from build123d import *

# Parameters (mm, degrees)
F1_DEPTH = 12.7
F2_DEPTH = 31.75
F3_R     = 12.7


with BuildPart() as f1:
    # F0 (on Right) → F1 (new body, symmetric)
    with BuildSketch(Plane.YZ):
        with BuildLine():
            ThreePointArc((31.059256, -22.06655), (36.29716, -11.581285), (38.1, 0))
            ThreePointArc((38.1, 0), (-11.489227, 36.326405), (-31.170744, -21.908782))
            Line((-31.170744, -21.908782), (31.059256, -21.908782))
            Line((31.059256, -21.908782), (31.059256, -22.06655))
        make_face()
        with BuildLine():
            Line((31.059256, -174.308782), (31.059256, -22.06655))
            ThreePointArc((31.059256, -22.06655), (17.476763, -33.855173), (0, -38.1))
            Line((0, -38.1), (-31.170744, -49.680229))
            Line((-31.170744, -49.680229), (-31.170744, -174.308782))
            Line((-31.170744, -174.308782), (31.059256, -174.308782))
        make_face()
        with BuildLine():
            Line((31.059256, -21.908782), (-31.170744, -21.908782))
            ThreePointArc((-31.170744, -21.908782), (-17.562537, -33.810757), (0, -38.1))
            ThreePointArc((0, -38.1), (17.476763, -33.855173), (31.059256, -22.06655))
            Line((31.059256, -22.06655), (31.059256, -21.908782))
        make_face()
    extrude(amount=F1_DEPTH, both=True)

    # F0 (on Right) → F2 (join, symmetric)
    with BuildSketch(Plane.YZ):
        with BuildLine():
            Line((31.059256, -174.308782), (31.059256, -22.06655))
            ThreePointArc((31.059256, -22.06655), (17.476763, -33.855173), (0, -38.1))
            Line((0, -38.1), (-31.170744, -49.680229))
            Line((-31.170744, -49.680229), (-31.170744, -174.308782))
            Line((-31.170744, -174.308782), (31.059256, -174.308782))
        make_face()
    extrude(amount=F2_DEPTH, both=True)

    # F3
    f3_edges = [f1.edges().sort_by_distance(p)[0] for p in [
        (31.75, -31.170744, -111.994506),
        (31.75, 31.059256, -98.187666),
        (-31.75, -31.170744, -111.994506),
        (-31.75, 31.059256, -98.187666),
    ]]
    fillet(f3_edges, radius=F3_R)


solid = f1.part
Read the model definition and answer for the solid it produces. Units are mm, in the model's axes. A direction names the side the tool comes from. Give positions to 0.01 mm unless a question says otherwise; leave off trailing zeros. Loops run counter-clockwise (first coordinate to the right, second up) from the corner with the lowest first, then second, coordinate; pieces in that order, holes last. Notation, with made-up numbers: (87.25, 52) -> (128.25, 52) arc R16 cw to (128.25, 80) -> close; hole circle Ø6 at (-38, 61.25). An arc over 180 degrees is marked (long way). Use a Markdown table: item, result.
Q1. Find the intervals of material crossed by line 1 along Y through (x, z) = (-14.5, -116); line 2 along X through (y, z) = (-34, 3.5); line 3 along Z through (x, y) = (-4.5, 1), in increasing order.
Solved:
| item | result |
|---|---|
| line 1 | y = -31.17 to 31.06 |
| line 2 | x = -12.7 to 12.7 |
| line 3 | z = -174.31 to 38.09 |
Q2. Section C-C, the plane y = -24 is taken. Determine the outline of the cut face in (x, z).
Solved:
| item | result |
|---|---|
| outline | (-30.48, -174.31) -> (30.48, -174.31) -> (30.48, -47.02) -> (-30.48, -47.02) -> close; (-12.7, -29.59) -> (12.7, -29.59) -> (12.7, 29.59) -> (-12.7, 29.59) -> close |
Q3. Section D-D, the plane y = 16 is taken. Determine the outline of the cut face in (x, z), then the cut area to 3 significant figures.
Solved:
| item | result |
|---|---|
| outline | (-31.75, -174.31) -> (31.75, -174.31) -> (31.75, -34.58) -> (12.7, -34.58) -> (12.7, 34.58) -> (-12.7, 34.58) -> (-12.7, -34.58) -> (-31.75, -34.58) -> close |
| area | 10,600 mm^2 |
Q4. A tool of negligible diameter and unlimited length cuts with its end or side. For faces 1 (the face through (-12.7, -1, 1)), 2 (the face through (0, -31.171, -111)), 3 (the face through (0, 31.059, -99)), 4 (the face through (12.7, -1, 1)), from which of +Z, -Z, +X, -X, +Y, -Y can it reach the whole face along a straight path? Write none if from no direction.
Solved:
| item | result |
|---|---|
| face 1 | +Z, -X, -Y |
| face 2 | -Z, +X, -X, -Y |
| face 3 | -Z, +X, -X, +Y |
| face 4 | +Z, +X, -Y |
Q5. Each of these flat-tipped pins is pushed along its axis until it touches: pin 1 (10 mm diameter, centred on x = -20.5, z = -75.5, fed in from -Y); pin 2 (1.5 mm diameter, centred on y = 22.5, z = -20.5, fed in from -X); pin 3 (19 mm diameter, centred on x = 5.5, z = -130, fed in from +Y). Where does it stop, or does it pass through?
Solved:
| item | result |
|---|---|
| pin 1 | stops at y = -31.17 |
| pin 2 | stops at x = -12.7 |
| pin 3 | stops at y = 31.06 |
Q6. Section B-B, the plane z = -128.5 is taken. Determine the outline of the cut face in (x, y), then the cut area to 3 significant figures.
Solved:
| item | result |
|---|---|
| outline | (-31.75, -18.47) arc R12.7 ccw to (-19.05, -31.17) -> (19.05, -31.17) arc R12.7 ccw to (31.75, -18.47) -> (31.75, 18.36) arc R12.7 ccw to (19.05, 31.06) -> (-19.05, 31.06) arc R12.7 ccw to (-31.75, 18.36) -> close |
| area | 3,810 mm^2 |
Q7. Determine the mould class of faces 5 (the face through (-27.93, -27.55, -110.54)), 6 (the face through (0, 0, -174.309)), 7 (the face through (-22.09, 17.7, -33.74)), 8 (the face through (0.44, -15.37, -43.81)) for opening direction Z: pulls with the +Z half, pulls with the -Z half, needs draft (parallel to the pull), parting line crosses it, or undercut.
Solved:
| item | result |
|---|---|
| face 5 | needs draft |
| face 6 | pulls with the -Z half |
| face 7 | pulls with the +Z half |
| face 8 | undercut |
Q8. Section A-A, the plane x = 1 is taken. Determine the outline of the cut face in (y, z), then the cut area to 3 significant figures.
Solved:
| item | result |
|---|---|
| outline | (-31.17, -174.31) -> (31.06, -174.31) -> (31.06, -22.07) arc R38.1 ccw to (38.1, 0) arc R38.1 ccw (long way) to (0, -38.1) -> (-31.17, -49.68) -> close |
| area | 13,000 mm^2 |
